For this review, take the finished solid that the model builds, in its own axes (mm). Face numbers are marked on the shaded views. A direction names the side the tool comes from. Coordinates: 2 decimals unless noted, no trailing zeros. Write each loop counter-clockwise with the first axis right and the second up, starting at its lowest first coordinate (ties: lowest second). Pieces come first, ordered by that corner, then holes. Notation, with made-up numbers: (8, -21.75) -> (61, -21.75) arc R21 ccw to (61, -1.75) -> close; hole circle Ø8 at (-10.5, 29). An arc over 180 degrees is marked (long way). Put each result on its own line as item: value. Start each with the question number.
Item 1: The part is to be moulded in two halves that separate along X. For the marked faces 1, 2 and 3, say which applies: +X half, -X half, draft (parallel to the pull), parting line (faces both ways), or undercut.
Item 2: Consider section D-D on x = 8. Give the boundary of the cut face in (y, z), and give its area (3 significant figures).
Item 3: Consider section B-B on z = 0. Give the boundary of the cut face in (x, y) (3 decimals).
Item 4: Insertion check: P1, Ø3, axis at x = 9.5, y = 9.5, coming from the +Z side; P2, Ø4, axis at y = 10.5, z = 5, coming from the -X side; P3, Ø11, axis at x = 0, z = 0, coming from the -Y side. Each pin has a flat end and moves straight along its axis. Give the tip position at first contact, or say it passes through.
Item 5: Consider section C-C on y = 4.25. Give the boundary of the cut face in (x, z) (3 decimals), and give its area (3 significant figures).
Item 6: Consider section A-A on x = 0. Give the boundary of the cut face in (y, z) (3 decimals), and give its area (3 significant figures).
Item 7: To check wall thickness, follow L1, parallel to X at y = 13, z = 0; L2, parallel to X at y = 4.5, z = 0.25; L3, parallel to Z at x = 0.75, y = 5.5. State the ranges of each line that lie inside material, in increasing order.
Item 8: For the marked faces 4, 5 and 6, list the 3-axis set-ups (+Z, -Z, +X, -X, +Y, -Y) from which the entire face can be reached by the end or side of a thin tool; tool diameter is ignored.
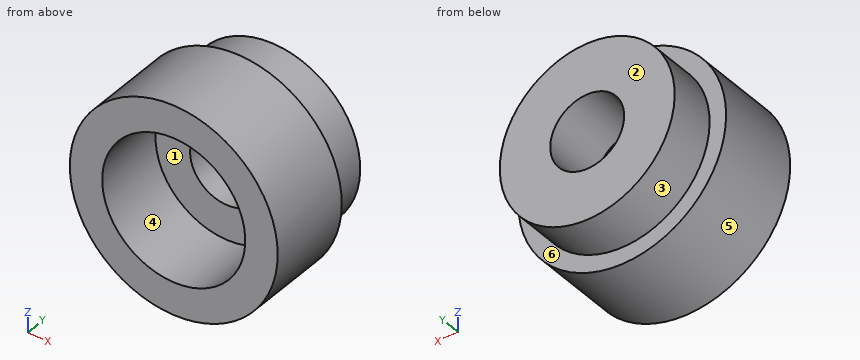
```python
from build123d import *

# Parameters (mm, degrees)
SKETCH1_R           = 11
SKETCH1_R_2         = 4.65
BOSS_EXTRUDE1_DEPTH = 17
SKETCH1_5_R         = 13.075
SKETCH1_5_R_2       = 11
BOSS_EXTRUDE2_DEPTH = 11
SKETCH2_R           = 9
CUT_EXTRUDE1_DEPTH  = 9.15


with BuildPart() as part:
    # Sketch1 → Boss-Extrude1 (new body)
    with BuildSketch(Plane(origin=(0, 0, 0), x_dir=(1, 0, 0), z_dir=(0, 1, 0))):
        with Locations(Location((0, 0, 0), (0, 0, 270))):
            Circle(SKETCH1_R)
        with Locations(Location((0, 0, 0), (0, 0, 270))):
            Circle(SKETCH1_R_2, mode=Mode.SUBTRACT)
    extrude(amount=BOSS_EXTRUDE1_DEPTH)

    # Sketch1_5 → Boss-Extrude2 (add)
    with BuildSketch(Plane(origin=(0, 0, 0), x_dir=(1, 0, 0), z_dir=(0, 1, 0))):
        with Locations(Location((0, 0, 0), (0, 0, 270))):
            Circle(SKETCH1_5_R)
        with Locations(Location((0, 0, 0), (0, 0, 270))):
            Circle(SKETCH1_5_R_2, mode=Mode.SUBTRACT)
    extrude(amount=BOSS_EXTRUDE2_DEPTH)

    # Sketch2 → Cut-Extrude1 (cut)
    with BuildSketch(Plane.XZ):
        with Locations(Location((0, 0, 0), (0, 0, 270))):
            Circle(SKETCH2_R)
    extrude(amount=-CUT_EXTRUDE1_DEPTH, mode=Mode.SUBTRACT)


solid = part.part
```
Return value:
1. face 1: undercut
1. face 2: draft
1. face 3: parting line
2. outline: (0, -10.34) -> (11, -10.34) -> (11, -7.55) -> (17, -7.55) -> (17, 7.55) -> (11, 7.55) -> (11, 10.34) -> (0, 10.34) -> (0, 4.12) -> (9.15, 4.12) -> (9.15, -4.12) -> (0, -4.12) -> close
2. area: 243 mm^2
3. outline: (-13.075, 0) -> (-9, 0) -> (-9, 9.15) -> (-4.65, 9.15) -> (-4.65, 17) -> (-11, 17) -> (-11, 11) -> (-13.075, 11) -> close; (4.65, 9.15) -> (9, 9.15) -> (9, 0) -> (13.075, 0) -> (13.075, 11) -> (11, 11) -> (11, 17) -> (4.65, 17) -> close
4. P1: z = 10.34
4. P2: x = -12.73
4. P3: y = 9.15
5. outline: circle Ø26.15 at (0, 0); hole circle Ø18 at (0, 0)
5. area: 283 mm^2
6. outline: (0, -13.075) -> (11, -13.075) -> (11, -11) -> (17, -11) -> (17, -4.65) -> (9.15, -4.65) -> (9.15, -9) -> (0, -9) -> close; (0, 9) -> (9.15, 9) -> (9.15, 4.65) -> (17, 4.65) -> (17, 11) -> (11, 11) -> (11, 13.075) -> (0, 13.075) -> close
6. area: 182 mm^2
7. L1: -11 to -4.65, 4.65 to 11
7. L2: -13.07 to -9, 9 to 13.07
7. L3: -13.05 to -8.97, 8.97 to 13.05
8. face 4: -Y
8. face 5: +Y, -Y
8. face 6: +Y
